Answer from the drawing. Dimensions are ordinates in mm from the lowest x, y and z of the part. A direction names the side the tool comes from. Give positions to 0.01 mm unless a question says otherwise; leave off trailing zeros. Loops run counter-clockwise (first coordinate to the right, second up) from the corner with the lowest first, then second, coordinate; pieces in that order, holes last. Notation, with made-up numbers: M -23,78.25 L 34,78.25 A18 cw 34,90.25 Z; hole C 63.5,-17.75 d10. An arc over 180 degrees is marked long. Use a Markdown table: item, result.
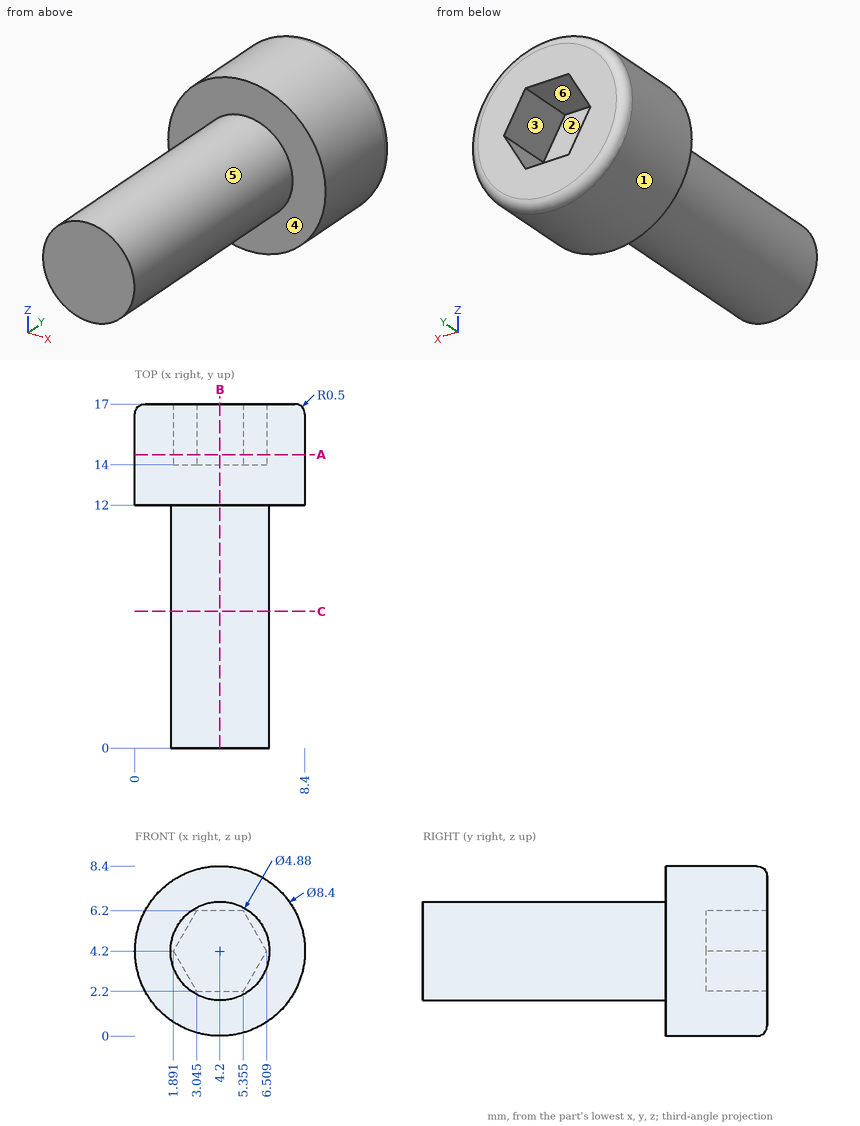
(1) Consider probe 1 along Y at (x, z) = (1.25, 3); probe 2 along Y at (x, z) = (2.75, 4); probe 3 along Z at (x, y) = (4.25, 11.5). Determine where each line is inside the solid, lowest interval first. Write a range as [from, to].
Entries:
| item | result |
|---|---|
| probe 1 | y = [12, 17] |
| probe 2 | y = [0, 14] |
| probe 3 | z = [1.76, 6.64] |
(2) A cutting plane is placed at B-B (x = 4.2). Write down the section's boundary in (y, z).
Entries:
| item | result |
|---|---|
| outline | M 0,1.76 L 12,1.76 L 12,0 L 16.5,0 A0.5 ccw 17,0.5 L 17,2.2 L 14,2.2 L 14,6.2 L 17,6.2 L 17,7.9 A0.5 ccw 16.5,8.4 L 12,8.4 L 12,6.64 L 0,6.64 Z |
(3) Given P1, Ø3, axis at x = 4, y = 2.5, coming from the -Z side; P2, Ø3, axis at x = 2, y = 7, coming from the -Z side; P3, Ø1.5, axis at x = 1.5, y = 15, coming from the +Z side, each flat-ended and moving along its own axis, determine where each tip first touches the part or whether it passes through.
Entries:
| item | result |
|---|---|
| P1 | stops at z = 1.76 |
| P2 | stops at z = 1.86 |
| P3 | stops at z = 7.92 |
(4) A cutting plane is placed at C-C (y = 6.75). Write down the section's boundary in (x, z), and give its area (3 significant figures).
Entries:
| item | result |
|---|---|
| outline | C 4.2,4.2 d4.88 |
| area | 18.7 mm² |
(5) The mould has two halves that part along X. Classify the marked faces 3, 4, 5 and 6: released by +X, released by -X, zero draft, split by the parting line, or undercut.
Entries:
| item | result |
|---|---|
| face 3 | undercut |
| face 4 | zero draft |
| face 5 | split by the parting line |
| face 6 | undercut |
(6) Which of the six approach directions +Z, -Z, +X, -X, +Y, -Y give full straight-line access (tool end or side, diameter ignored) to the marked faces 1 and 2?
Entries:
| item | result |
|---|---|
| face 1 | +Y, -Y |
| face 2 | +Y |
(7) A cutting plane is placed at A-A (y = 14.5). Write down the section's boundary in (x, z) (1 decimal).
Entries:
| item | result |
|---|---|
| outline | C 4.2,4.2 d8.4; hole M 1.9,4.2 L 3,2.2 L 5.4,2.2 L 6.5,4.2 L 5.4,6.2 L 3,6.2 Z |
